Read the model definition and answer for the solid it produces. Units are mm, in the model's axes. A direction names the side the tool comes from. Round coordinates to 2 decimals unless told otherwise and drop trailing zeros. Order: outer loops, then holes, each group sorted by start corner. A loop starts at its lowest first (then second) coordinate and runs counter-clockwise, first axis right, second up. Notation, with made-up numbers: (-9.5, 51.5) - (-2.5, 51.5) arc R27 cw to (-2.5, 71.5) - close; hole circle Ø3 at (-7.75, -1). An arc over 180 degrees is marked (long way). Answer as a JSON object with one key per item and string values. Group by question number.
Q1. The mould has two halves that part along Y. Classify faces 1 (the flat face through (-20, 0, 10)), 2 (the flat face through (-16, 12.5, 10)), 3 (the flat face through (0, -12.5, 5)), 4 (the flat face through (8.768, -1.486, 9.86)): pulls with the +Y half, pulls with the -Y half, needs draft (parallel to the pull), parting line crosses it, or undercut.
Q2. A cutting plane is placed at C-C on z = 10. Determine the outline of the cut face in (x, y), and give its area (3 significant figures).
Q3. Consider line 1 (Z direction, x = 0, y = -7.5); line 2 (X direction, y = 6, z = 13); line 3 (Y direction, x = 5, z = 11). Determine where each line is inside the solid, lowest interval first.
Q4. A tool of negligible diameter and unlimited length cuts with its end or side. For faces 5 (the flat face through (-6.6, 6, 10)), 6 (the flat face through (8, 4, 10)), 7 (the flat face through (0, -3, 20)), from which of +Z, -Z, +X, -X, +Y, -Y can it reach the whole face along a straight path? Write none if from no direction.
Q5. A cutting plane is placed at B-B on y = 4.25. Determine the outline of the cut face in (x, z), and give its area (3 significant figures).
Q6. A cutting plane is placed at D-D on z = 2. Determine the outline of the cut face in (x, y).
Q7. A cutting plane is placed at A-A on x = 0. Determine the outline of the cut face in (y, z), and give its area (3 significant figures).
Q8. Given pin 1 Ø4 at (x, z) = (0, 10) entering from -Y; pin 2 Ø1.5 at (x, z) = (7, 13.5) entering from +Y, each flat-ended and moving along its own axis, determine where each tip first touches the part or whether it passes through.
```python
from build123d import *

# Parameters (mm, degrees)
SKETCH_1_W               = 40
SKETCH_1_H               = 25
EXTRUDE_1_DEPTH          = 20
CUT_EXTRUDE_1_DEPTH      = 1
CUT_EXTRUDE_1_DEPTH_BACK = 20
HOLE_WIZARD_M6_1_D       = 5
HOLE_WIZARD_M6_1_DEPTH   = 18
HOLE_WIZARD_M6_1_TIP     = 1.502151548


with BuildPart() as part:
    # 草图1 → 凸台-拉伸1 (new body)
    with BuildSketch(Plane.XY):
        Rectangle(SKETCH_1_W, SKETCH_1_H)
    extrude(amount=EXTRUDE_1_DEPTH)

    # 草图2 → 切除-拉伸1 (cut, two sides)
    with BuildSketch(Plane(origin=(0, 0, 0), x_dir=(-1, 0, 0), z_dir=(0, 0, -1))) as cut_extrude_1_sk:
        Polygon((-78.390332326, 76.715154385), (-12.5, 12.5), (-6.6, 6.75), (-6.6, 5.75), (-10, 1.5), (-10, -0.5), (-7.5, -2.5), (7.5, -2.5), (10, -0.5), (10, 1.5), (6.6, 5.75), (6.6, 6.75), (12.5, 12.5), (78.390332326, 76.715154385), (78.390332326, 260.727349054), (-78.390332326, 260.727349054), align=None)
    extrude(amount=CUT_EXTRUDE_1_DEPTH, mode=Mode.SUBTRACT)
    extrude(cut_extrude_1_sk.sketch, amount=-CUT_EXTRUDE_1_DEPTH_BACK, mode=Mode.SUBTRACT)

    # M6 螺纹孔1
    with Locations(Plane(origin=(0, -12.5, 0), x_dir=(-1, 0, 0), z_dir=(0, -1, 0))):
        with Locations((0, -10)):
            Hole(HOLE_WIZARD_M6_1_D / 2, depth=HOLE_WIZARD_M6_1_DEPTH)
            with Locations((0, 0, -(HOLE_WIZARD_M6_1_DEPTH + HOLE_WIZARD_M6_1_TIP / 2))):  # 118° drill point
                Cone(0, HOLE_WIZARD_M6_1_D / 2, HOLE_WIZARD_M6_1_TIP, mode=Mode.SUBTRACT)


solid = part.part
```
Result set:
{
 "1": {"face 1": "needs draft", "face 2": "pulls with the +Y half", "face 3": "pulls with the -Y half", "face 4": "undercut"},
 "2": {"outline": "(-20, -12.5) - (-2.5, -12.5) - (-2.5, -2.5) - (-7.5, -2.5) - (-10, -0.5) - (-10, 1.5) - (-6.6, 5.75) - (-6.6, 6.75) - (-12.5, 12.5) - (-20, 12.5) - close; (2.5, -12.5) - (20, -12.5) - (20, 12.5) - (12.5, 12.5) - (6.6, 6.75) - (6.6, 5.75) - (10, 1.5) - (10, -0.5) - (7.5, -2.5) - (2.5, -2.5) - close", "area": "681 mm²"},
 "3": {"line 1": "z = 0 to 7.5, 12.5 to 20", "line 2": "x = -20 to -6.6, 6.6 to 20", "line 3": "y = -12.5 to -2.5"},
 "4": {"face 5": "+Z, -Z, +Y", "face 6": "+Z, -Z", "face 7": "+Z, +X, -X, +Y, -Y"},
 "5": {"outline": "(-20, 0) - (-7.8, 0) - (-7.8, 20) - (-20, 20) - close; (7.8, 0) - (20, 0) - (20, 20) - (7.8, 20) - close", "area": "488 mm²"},
 "6": {"outline": "(-20, -12.5) - (20, -12.5) - (20, 12.5) - (12.5, 12.5) - (6.6, 6.75) - (6.6, 5.75) - (10, 1.5) - (10, -0.5) - (7.5, -2.5) - (-7.5, -2.5) - (-10, -0.5) - (-10, 1.5) - (-6.6, 5.75) - (-6.6, 6.75) - (-12.5, 12.5) - (-20, 12.5) - close"},
 "7": {"outline": "(-12.5, 0) - (-2.5, 0) - (-2.5, 7.5) - (-12.5, 7.5) - close; (-12.5, 12.5) - (-2.5, 12.5) - (-2.5, 20) - (-12.5, 20) - close", "area": "150 mm²"},
 "8": {"pin 1": "passes through", "pin 2": "stops at y = 7.87"}
}
